Autodesk Inventor part; units mm, degrees
ref_plane "YZ Plane" through (0, 0, 0) normal (1, 0, 0) x (0, 1, 0)
ref_plane "XZ Plane" through (0, 0, 0) normal (0, 1, 0) x (-1, 0, 0)
ref_plane "XY Plane" through (0, 0, 0) normal (0, 0, 1) x (1, 0, 0)
sketch "Sketch2" plane through (0, 0, 0) normal (0, 0, 1) x (1, 0, 0)
  line L0 (-4.7625, -4.7625) -> (4.7625, -4.7625)
  line L1 (4.7625, -4.7625) -> (4.7625, 4.7625)
  line L2 (4.7625, 4.7625) -> (-4.7625, 4.7625)
  line L3 (-4.7625, 4.7625) -> (-4.7625, -4.7625)
  line L4 (-4.7625, -4.7625) -> (4.7625, 4.7625) construction
  line L5 (4.7625, -4.7625) -> (-4.7625, 4.7625) construction
  line L6 (-4.7625, 4.7625) -> (4.7625, -4.7625)
  line L7 (4.7625, -4.7625) -> (-0.3562, -9.8812)
  line L8 (-0.3562, -9.8812) -> (-9.8812, -0.3562)
  line L9 (-9.8812, -0.3562) -> (-4.7625, 4.7625)
  line L10 (-9.8812, -0.3562) -> (-9.8812, -9.8812)
  line L11 (-9.8812, -9.8812) -> (-0.3562, -9.8812)
  line L12 (-0.3562, -9.8812) -> (-0.3562, -0.3562)
  line L13 (-0.3562, -0.3562) -> (-9.8812, -0.3562)
  line L14 (-9.8812, -0.3562) -> (-0.3562, -9.8812) construction
  line L15 (-9.8812, -9.8812) -> (-0.3562, -0.3562) construction
  point P0 (0, 0)
  point P1 (-5.1187, -5.1187)
  point P2 (-5.1187, -5.1187)
  dimension "clip_edge" = 9.525
  dimension "d1" = 9.525
  dimension "d2" = 7.239
  dimension "d39" = 9.525
  dimension "d40" = 9.525
extrude "Extrusion1" add sketch "Sketch2" along normal blind 1.5875
sketch "Sketch3" plane through (0, 0, 0) normal (0, 0, -1) x (-1, 0, 0)
  line L0 (6.1855, -6.1855) -> (-0.1905, 0.1905)
  line L1 (0.3562, -9.8812) -> (-4.7625, -4.7625) construction
  line L2 (-4.7625, 4.7625) -> (5.1187, -5.1187) construction
  line L3 (9.8812, -0.3562) -> (0.3562, -9.8812) construction
  line L4 (-4.7625, 4.7625) -> (4.7625, 4.7625)
  line L5 (6.1855, -6.1855) -> (-0.1905, 0.1905) construction
  line L6 (7.2631, -5.1079) -> (0.8871, 1.2681)
  line L7 (-1.2681, -0.8871) -> (5.1079, -7.2631)
  arc A0 (5.1079, -7.2631) -> (7.2631, -5.1079) centre (6.1855, -6.1855) ccw
  arc A1 (0.8871, 1.2681) -> (-1.2681, -0.8871) centre (-0.1905, 0.1905) ccw
  point P0 (0, 0)
  point P1 (2.9975, -2.9975)
  dimension "d5" = 9.017
  dimension "d6" = 4.572
  dimension "d31" = 3.048
extrude "Extrusion7" cut sketch "Sketch3" against normal through all
fillet "Fillet13" radius 1.5875 6 edges at (-4.7625, 4.7625, 0.7937) (-9.8812, -0.3562, 0.7937) (-9.8812, -9.8812, 0.7937) (4.7625, -4.7625, 0.7937) (4.7625, 4.7625, 0.7937) (-0.3562, -9.8812, 0.7937)
equation "\"d1\" = clip_edge"
properties part number "hph_D_001"
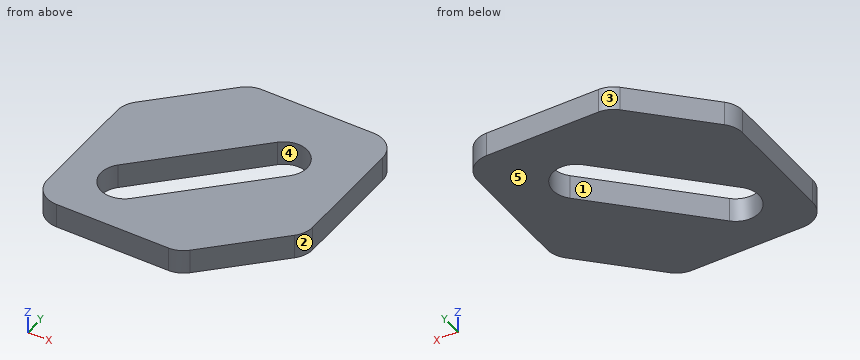
Read the model definition and answer for the solid it produces. Units are mm, in the model's axes. Face numbers are marked on the shaded views. A direction names the side the tool comes from. Coordinates: 2 decimals unless noted, no trailing zeros. Write each loop counter-clockwise with the first axis right and the second up, starting at its lowest first coordinate (ties: lowest second). Pieces come first, ordered by that corner, then holes. Notation, with made-up numbers: M 80.25,-11.75 L 117.25,-11.75 A17 cw 117.25,4.25 Z; hole C 11,31 d10. An arc over 180 degrees is marked long. Use a Markdown table: item, result.
Q1. This flat-tipped pin is pushed along its axis until it touches: pin 1 Ø5 at (x, y) = (2, 0.5) entering from -Z. Where does it stop, or does it pass through?
Answer block:
| item | result |
|---|---|
| pin 1 | stops at z = 0 |
Q2. The part is cut by section C-C, the plane x = -6.25. Write down the section's boundary in (y, z) (1 decimal), then the cut area to 3 significant figures.
Answer block:
| item | result |
|---|---|
| outline | M -9.9,0 L -7.7,0 L -7.7,1.6 L -9.9,1.6 Z; M -4.1,0 L 3.3,0 L 3.3,1.6 L -4.1,1.6 Z |
| area | 15.1 mm2 |
Q3. Straight lines are drawn through the part: L1, parallel to X at y = -2.75, z = 0.6; L2, parallel to Y at x = -5.75, z = 1.2 (3 decimals); L3, parallel to Y at x = -4, z = 0.8. For each, find the intervals that lie inside material, in ascending order. Write a range as [from, to].
Answer block:
| item | result |
|---|---|
| L1 | x = [-9.88, -4.91], [-0.59, 4.76] |
| L2 | y = [-9.881, -7.646], [-3.595, 3.775] |
| L3 | y = [-9.88, -6.16], [-1.84, 4.76] |
Q4. The part is cut by section B-B, the plane z = 1.3. Write down the section's boundary in (x, y) (1 decimal), then the cut area to 3 significant figures.
Answer block:
| item | result |
|---|---|
| outline | M -9.9,-8.3 A1.6 ccw -8.3,-9.9 L -1,-9.9 A1.6 ccw 0.1,-9.4 L 4.3,-5.2 A1.6 ccw 4.8,-4.1 L 4.8,3.2 A1.6 ccw 3.2,4.8 L -4.1,4.8 A1.6 ccw -5.2,4.3 L -9.4,0.1 A1.6 ccw -9.9,-1 Z; hole M -7.3,-5.1 A1.5 ccw -5.1,-7.3 L 1.3,-0.9 A1.5 ccw -0.9,1.3 Z |
| area | 152 mm2 |
Q5. The part is cut by section D-D, the plane y = 2. Write down the section's boundary in (x, z) (1 decimal).
Answer block:
| item | result |
|---|---|
| outline | M -7.5,0 L 4.8,0 L 4.8,1.6 L -7.5,1.6 Z |
Q6. The part is cut by section A-A, the plane y = -5.5. Write down the section's boundary in (x, z) (1 decimal), then the cut area to 3 significant figures.
Answer block:
| item | result |
|---|---|
| outline | M -9.9,0 L -7.5,0 L -7.5,1.6 L -9.9,1.6 Z; M -3.3,0 L 4,0 L 4,1.6 L -3.3,1.6 Z |
| area | 15.4 mm2 |
Q7. Determine the mould class of the marked faces 3, 4 and 5 for opening direction X: released by +X, released by -X, zero draft, split by the parting line, or undercut.
Answer block:
| item | result |
|---|---|
| face 3 | released by -X |
| face 4 | undercut |
| face 5 | zero draft |
Q8. Which of the six approach directions +Z, -Z, +X, -X, +Y, -Y give full straight-line access (tool end or side, diameter ignored) to the marked faces 1 and 2?
Answer block:
| item | result |
|---|---|
| face 1 | +Z, -Z |
| face 2 | +Z, -Z, +X, -Y |
